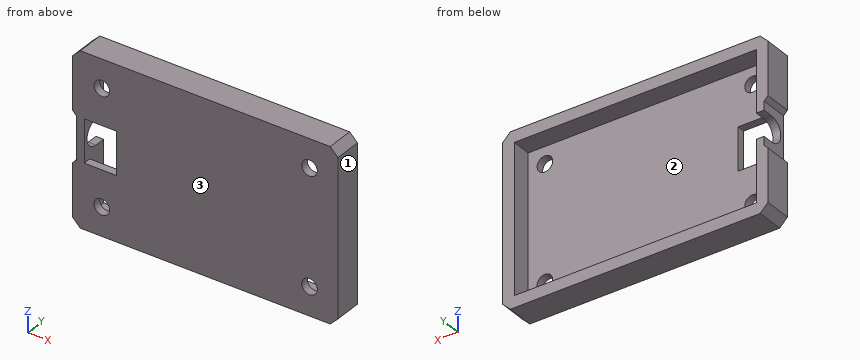
from build123d import *

# Parameters (mm, degrees)
BOSS_EXTRUDE1_DEPTH = 5
SKETCH2_W           = 68
SKETCH2_H           = 44
BOSS_EXTRUDE2_DEPTH = 2
SKETCH3_W           = 11
SKETCH3_H           = 2
CUT_EXTRUDE1_DEPTH  = 11.2
CHAMFER1_SIZE       = 1
SKETCH4_R           = 2
CUT_EXTRUDE2_DEPTH  = 10
SKETCH6_W           = 2
SKETCH6_H           = 7
BOSS_EXTRUDE3_DEPTH = 20
CUT_EXTRUDE3_DEPTH  = 5
CHAMFER2_SIZE       = 2


with BuildPart() as part:
    # Sketch1 → Boss-Extrude1 (new body)
    with BuildSketch(Plane(origin=(0, 0, 0), x_dir=(1, 0, 0), z_dir=(0, 1, 0))):
        Polygon((-33.284090909, -14.318181818), (-33.284090909, -27.818181818), (28.715909091, -27.818181818), (28.715909091, 10.181818182), (-33.284090909, 10.181818182), (-33.284090909, -3.318181818), (-36.284090909, -3.318181818), (-36.284090909, 13.181818182), (31.715909091, 13.181818182), (31.715909091, -30.818181818), (-36.284090909, -30.818181818), (-36.284090909, -14.318181818), align=None)
    extrude(amount=BOSS_EXTRUDE1_DEPTH)

    # Sketch2 → Boss-Extrude2 (add)
    with BuildSketch(Plane.XZ):
        with Locations((-2.284090909, 8.818181818)):
            Rectangle(SKETCH2_W, SKETCH2_H)
    extrude(amount=BOSS_EXTRUDE2_DEPTH)

    # Sketch3 → Cut-Extrude1 (cut)
    with BuildSketch(Plane.ZY.offset(36.284090909)):
        with Locations((8.818181818, -1)):
            Rectangle(SKETCH3_W, SKETCH3_H)
    extrude(amount=-CUT_EXTRUDE1_DEPTH, mode=Mode.SUBTRACT)

    # Chamfer1
    chamfer1_edges = [part.edges().sort_by_distance(p)[0] for p in [
        (-36.284090909, 1.5, 3.318181818),
        (-36.284090909, 1.5, 14.318181818),
    ]]
    chamfer(chamfer1_edges, length=CHAMFER1_SIZE)

    # Sketch4 → Cut-Extrude2 (cut)
    with BuildSketch(Plane(origin=(0, 0, 0), x_dir=(1, 0, 0), z_dir=(0, 1, 0))):
        with Locations(Location((24.415909091, 5.881818182, 0), (0, 0, 270))):
            Circle(SKETCH4_R)
        with Locations(Location((24.415909091, -23.518181818, 0), (0, 0, 270))):
            Circle(SKETCH4_R)
        with Locations(Location((-28.784090909, -23.518181818, 0), (0, 0, 270))):
            Circle(SKETCH4_R)
        with Locations(Location((-28.784090909, 5.881818182, 0), (0, 0, 270))):
            Circle(SKETCH4_R)
    extrude(amount=-CUT_EXTRUDE2_DEPTH, mode=Mode.SUBTRACT)

    # Sketch6 → Boss-Extrude3 (add)
    with BuildSketch(Plane(origin=(0, 0, 14.318181818), x_dir=(-1, 0, 0), z_dir=(0, 0, -1))):
        with Locations((34.284090909, 1.5)):
            Rectangle(SKETCH6_W, SKETCH6_H)
    extrude(amount=BOSS_EXTRUDE3_DEPTH)

    # Sketch7 → Cut-Extrude3 (cut)
    with BuildSketch(Plane.ZY.offset(35.284090909)):
        with BuildLine():
            Line((5.568181818, 2.25), (5.568181818, 5))
            Line((5.568181818, 5), (12.068181818, 5))
            Line((12.068181818, 5), (12.068181818, 2.25))
            ThreePointArc((12.068181818, 2.25), (8.818181818, -1), (5.568181818, 2.25))
        make_face()
    extrude(amount=-CUT_EXTRUDE3_DEPTH, mode=Mode.SUBTRACT)

    # Chamfer2
    chamfer2_edges = [part.edges().sort_by_distance(p)[0] for p in [
        (-36.284090909, 1.5, -13.181818182),
        (31.715909091, 1.5, -13.181818182),
        (31.715909091, 1.5, 30.818181818),
        (-36.284090909, 1.5, 30.818181818),
    ]]
    chamfer(chamfer2_edges, length=CHAMFER2_SIZE)


solid = part.part
Work out the finished part from the listing and answer in its coordinate system (mm). Face numbers are marked on the shaded views. Round coordinates to 2 decimals unless told otherwise and drop trailing zeros. Loops run counter-clockwise (first coordinate to the right, second up) from the corner with the lowest first, then second, coordinate; pieces in that order, holes last. Notation, with made-up numbers: M -39,-4.5 L -13,-4.5 A16 cw -13,21.5 Z; hole C 85,-11.75 d9. An arc over 180 degrees is marked long. One line per question, with ' | ' between items. Start each with the question number.
(1) Find the intervals of material crossed by line 1 (Z direction, x = 11.5, y = 3.5); line 2 (X direction, y = 0.5, z = 22.5); line 3 (Y direction, x = -3, z = 19), in increasing order.
(2) A cutting plane is placed at D-D on z = -2. Write down the section's boundary in (x, y).
(3) A cutting plane is placed at A-A on z = -7. Write down the section's boundary in (x, y).
(4) Flat-ended cylindrical pins translate along their axes: pin 1 Ø1 at (y, z) = (2.5, 5) entering from -X; pin 2 Ø6 at (x, z) = (12.5, -2) entering from +Y; pin 3 Ø2 at (y, z) = (2.5, 11) entering from -X. Find the tip coordinate at first contact, or state that the pin passes through.
(5) For a pull along X with two mould halves and no side action, classify the marked faces 1, 2 and 3 as released by +X, released by -X, zero draft, split by the parting line, or undercut.
(6) A cutting plane is placed at B-B on y = 4. Write down the section's boundary in (x, z), plus the area to 3 significant figures.
(7) A cutting plane is placed at C-C on x = -17.5. Write down the section's boundary in (y, z).
Geometry check:
1) line 1: z = -13.18 to -10.18, 27.82 to 30.82 | line 2: x = -36.28 to -33.28, 28.72 to 31.72 | line 3: y = -2 to 0
2) outline: M -36.28,-2 L 31.72,-2 L 31.72,5 L 28.72,5 L 28.72,0 L -33.28,0 L -33.28,5 L -36.28,5 Z
3) outline: M -36.28,-2 L -30.44,-2 L -30.44,0 L -33.28,0 L -33.28,5 L -36.28,5 Z; M -27.13,-2 L 22.76,-2 L 22.76,0 L -27.13,0 Z; M 26.07,-2 L 31.72,-2 L 31.72,5 L 28.72,5 L 28.72,0 L 26.07,0 Z
4) pin 1: stops at x = -35.28 | pin 2: stops at y = 0 | pin 3: stops at x = 28.72
5) face 1: released by +X | face 2: undercut | face 3: zero draft
6) outline: M -36.28,-11.18 L -34.28,-13.18 L 29.72,-13.18 L 31.72,-11.18 L 31.72,28.82 L 29.72,30.82 L -34.28,30.82 L -36.28,28.82 L -36.28,15.32 L -35.28,14.32 L -35.28,12.07 L -33.28,12.07 L -33.28,27.82 L 28.72,27.82 L 28.72,-10.18 L -33.28,-10.18 L -33.28,5.57 L -35.28,5.57 L -35.28,3.32 L -36.28,2.32 Z | area: 603 mm²
7) outline: M -2,-13.18 L 5,-13.18 L 5,-10.18 L 0,-10.18 L 0,27.82 L 5,27.82 L 5,30.82 L -2,30.82 Z
